Read the model definition and answer for the solid it produces. Units are mm, in the model's axes. A direction names the side the tool comes from. Give positions to 0.01 mm unless a question says otherwise; leave off trailing zeros. Loops run counter-clockwise (first coordinate to the right, second up) from the corner with the lowest first, then second, coordinate; pieces in that order, holes last. Notation, with made-up numbers: (33.25, 8.25) - (74.25, 8.25) arc R6 ccw to (74.25, 15.25) - close; hole circle Ø1 at (-20, 57.25). An arc over 180 degrees is marked (long way). Use a Markdown table: item, result. Add a question column.
Item 1: Which of the six approach directions +Z, -Z, +X, -X, +Y, -Y give full straight-line access (tool end or side, diameter ignored) to faces 1 (the face through (8, -12, -8.5)), 2 (the face through (34, -16, 0)), 3 (the face through (22, -13.75, 0)), 4 (the face through (0, 6, -10)), 5 (the face through (-32, -13.75, 0))?
Item 2: Consider probe 1 along X at (y, z) = (-16.85, 0); probe 2 along X at (y, z) = (-5.5, -2.25); probe 3 along Z at (x, y) = (6.5, 7.5). Determine where each line is inside the solid, lowest interval first. Write a range as [from, to].
Item 3: A cutting plane is placed at B-B (z = 0). Give the number of separate pieces and of enclosed holes in the cut face, plus the area to 3 significant figures.
Item 4: A cutting plane is placed at A-A (x = 6.91). Determine the outline of the cut face in (y, z) (3 decimals).
Item 5: For a pull along Z with two mould halves and no side action, classify faces 6 (the face through (0, 0, -11)), 7 (the face through (-4, -5.25, 0)), 8 (the face through (20, 2, 0)), 9 (the face through (-24.47, -16.84, -0.33)) as +Z half, -Z half, draft (parallel to the pull), parting line (faces both ways), or undercut.
Item 6: Each of these flat-tipped pins is pushed along its axis until it touches: P1, Ø10, axis at x = 5.5, y = -11, coming from the +Z side; P2, Ø1.5, axis at y = -4.5, z = -0.5, coming from the +X side; P3, Ø4.5, axis at y = -10.5, z = -0.5, coming from the -X side; P4, Ø7.5, axis at x = -29, z = 0, coming from the +Y side. Where does it stop, or does it pass through?
Item 7: A cutting plane is placed at D-D (x = -27). Determine the outline of the cut face in (y, z), plus the area to 3 significant figures.
Item 8: A cutting plane is placed at C-C (y = 14). Determine the outline of the cut face in (x, z), plus the area to 3 significant figures.
from build123d import *

# Parameters (mm, degrees)
SKETCH1_W           = 14
SKETCH1_H           = 22
SKETCH1_R           = 4.6
SKETCH1_R_2         = 2.55
SKETCH1_W_2         = 40
SKETCH1_W_3         = 12
SKETCH1_H_2         = 9.2
BOSS_EXTRUDE1_DEPTH = 17.75
CUT_EXTRUDE1_START  = -13.75
SKETCH1_5_W         = 14
SKETCH1_5_H         = 22
SKETCH1_5_R         = 4.6
SKETCH1_5_R_2       = 2.55
CUT_EXTRUDE1_DEPTH  = 31.5
CUT_EXTRUDE2_START  = -15.95
SKETCH1_6_R         = 4.6
SKETCH1_6_R_2       = 2.55
CUT_EXTRUDE2_DEPTH  = 2.2
CUT_EXTRUDE3_START  = 17.75
SKETCH1_7_W         = 12
SKETCH1_7_H         = 9.2
CUT_EXTRUDE3_DEPTH  = 23
CUT_EXTRUDE4_START  = -5.25
SKETCH1_8_W         = 12
SKETCH1_8_H         = 9.2
CUT_EXTRUDE4_DEPTH  = 9
CUT_EXTRUDE5_REACH  = 46.216
SKETCH2_R           = 2
SKETCH2_3_R         = 4.125
CUT_EXTRUDE6_DEPTH  = 2.5


with BuildPart() as part:
    # Sketch1 → Boss-Extrude1 (new, symmetric)
    # profile 1 of 7: a face of its own
    with BuildSketch(Plane(origin=(0, 0, 0), x_dir=(1, 0, 0), z_dir=(0, 1, 0))):
        with Locations((-27, 0)):
            Rectangle(SKETCH1_W, SKETCH1_H)
        with Locations((-27, 0)):
            Circle(SKETCH1_R, mode=Mode.SUBTRACT)
    # profile 2 of 7: a face of its own
    with BuildSketch(Plane(origin=(0, 0, 0), x_dir=(1, 0, 0), z_dir=(0, 1, 0))):
        with Locations((-27, 0)):
            Circle(SKETCH1_R)
        with Locations(Location((-27, 0, 0), (0, 0, 270))):
            Circle(SKETCH1_R_2, mode=Mode.SUBTRACT)
    # profile 3 of 7: a face of its own
    with BuildSketch(Plane(origin=(0, 0, 0), x_dir=(1, 0, 0), z_dir=(0, 1, 0))):
        Rectangle(SKETCH1_W_2, SKETCH1_H)
        with BuildLine():
            Line((11.854501341, -10), (-11.854501341, -10))
            ThreePointArc((-11.854501341, -10), (-18.86, 0), (-11.854501341, 10))
            Line((-11.854501341, 10), (11.854501341, 10))
            ThreePointArc((11.854501341, 10), (18.86, 0), (11.854501341, -10))
        make_face(mode=Mode.SUBTRACT)
    # profile 4 of 7: a face of its own
    with BuildSketch(Plane(origin=(0, 0, 0), x_dir=(1, 0, 0), z_dir=(0, 1, 0))):
        with BuildLine():
            ThreePointArc((11.854501341, 10), (18.86, 0), (11.854501341, -10))
            Line((11.854501341, -10), (-11.854501341, -10))
            ThreePointArc((-11.854501341, -10), (-18.86, 0), (-11.854501341, 10))
            Line((-11.854501341, 10), (11.854501341, 10))
        make_face()
        with Locations((6.92918915, 0)):
            Rectangle(SKETCH1_W_3, SKETCH1_H_2, mode=Mode.SUBTRACT)
    # profile 5 of 7: a face of its own
    with BuildSketch(Plane(origin=(0, 0, 0), x_dir=(1, 0, 0), z_dir=(0, 1, 0))):
        with Locations((6.92918915, 0)):
            Rectangle(SKETCH1_W_3, SKETCH1_H_2)
    # profile 6 of 7: a face of its own
    with BuildSketch(Plane(origin=(0, 0, 0), x_dir=(1, 0, 0), z_dir=(0, 1, 0))):
        with Locations((27, 0)):
            Rectangle(SKETCH1_W, SKETCH1_H)
        with Locations((27, 0)):
            Circle(SKETCH1_R, mode=Mode.SUBTRACT)
    # profile 7 of 7: a face of its own
    with BuildSketch(Plane(origin=(0, 0, 0), x_dir=(1, 0, 0), z_dir=(0, 1, 0))):
        with Locations((27, 0)):
            Circle(SKETCH1_R)
        with Locations(Location((27, 0, 0), (0, 0, 270))):
            Circle(SKETCH1_R_2, mode=Mode.SUBTRACT)
    extrude(amount=BOSS_EXTRUDE1_DEPTH, both=True)

    # Sketch1<5> → Cut-Extrude1 (cut)
    # profile 1 of 4: a face of its own
    with BuildSketch(Plane(origin=(0, 0, 0), x_dir=(1, 0, 0), z_dir=(0, 1, 0)).offset(CUT_EXTRUDE1_START)):
        with Locations((-27, 0)):
            Rectangle(SKETCH1_5_W, SKETCH1_5_H)
        with Locations((-27, 0)):
            Circle(SKETCH1_5_R, mode=Mode.SUBTRACT)
    # profile 2 of 4: a face of its own
    with BuildSketch(Plane(origin=(0, 0, 0), x_dir=(1, 0, 0), z_dir=(0, 1, 0)).offset(CUT_EXTRUDE1_START)):
        with Locations((27, 0)):
            Rectangle(SKETCH1_5_W, SKETCH1_5_H)
        with Locations((27, 0)):
            Circle(SKETCH1_5_R, mode=Mode.SUBTRACT)
    # profile 3 of 4: a face of its own
    with BuildSketch(Plane(origin=(0, 0, 0), x_dir=(1, 0, 0), z_dir=(0, 1, 0)).offset(CUT_EXTRUDE1_START)):
        with Locations((-27, 0)):
            Circle(SKETCH1_5_R)
        with Locations(Location((-27, 0, 0), (0, 0, 270))):
            Circle(SKETCH1_5_R_2, mode=Mode.SUBTRACT)
    # profile 4 of 4: a face of its own
    with BuildSketch(Plane(origin=(0, 0, 0), x_dir=(1, 0, 0), z_dir=(0, 1, 0)).offset(CUT_EXTRUDE1_START)):
        with Locations((27, 0)):
            Circle(SKETCH1_5_R)
        with Locations(Location((27, 0, 0), (0, 0, 270))):
            Circle(SKETCH1_5_R_2, mode=Mode.SUBTRACT)
    extrude(amount=CUT_EXTRUDE1_DEPTH, mode=Mode.SUBTRACT)

    # Sketch1<6> → Cut-Extrude2 (cut)
    # profile 1 of 2: a face of its own
    with BuildSketch(Plane(origin=(0, 0, 0), x_dir=(1, 0, 0), z_dir=(0, 1, 0)).offset(CUT_EXTRUDE2_START)):
        with Locations(Location((-27, 0, 0), (0, 0, 270))):
            Circle(SKETCH1_6_R)
        with Locations(Location((-27, 0, 0), (0, 0, 270))):
            Circle(SKETCH1_6_R_2, mode=Mode.SUBTRACT)
    # profile 2 of 2: a face of its own
    with BuildSketch(Plane(origin=(0, 0, 0), x_dir=(1, 0, 0), z_dir=(0, 1, 0)).offset(CUT_EXTRUDE2_START)):
        with Locations(Location((27, 0, 0), (0, 0, 270))):
            Circle(SKETCH1_6_R)
        with Locations(Location((27, 0, 0), (0, 0, 270))):
            Circle(SKETCH1_6_R_2, mode=Mode.SUBTRACT)
    extrude(amount=CUT_EXTRUDE2_DEPTH, mode=Mode.SUBTRACT)

    # Sketch1<7> → Cut-Extrude3 (cut)
    # profile 1 of 2: a face of its own
    with BuildSketch(Plane(origin=(0, 0, 0), x_dir=(1, 0, 0), z_dir=(0, 1, 0)).offset(CUT_EXTRUDE3_START)):
        with BuildLine():
            ThreePointArc((11.854501341, 10), (18.86, 0), (11.854501341, -10))
            Line((11.854501341, -10), (-11.854501341, -10))
            ThreePointArc((-11.854501341, -10), (-18.86, 0), (-11.854501341, 10))
            Line((-11.854501341, 10), (11.854501341, 10))
        make_face()
        with Locations((6.92918915, 0)):
            Rectangle(SKETCH1_7_W, SKETCH1_7_H, mode=Mode.SUBTRACT)
    # profile 2 of 2: a face of its own
    with BuildSketch(Plane(origin=(0, 0, 0), x_dir=(1, 0, 0), z_dir=(0, 1, 0)).offset(CUT_EXTRUDE3_START)):
        with Locations((6.92918915, 0)):
            Rectangle(SKETCH1_7_W, SKETCH1_7_H)
    extrude(amount=-CUT_EXTRUDE3_DEPTH, mode=Mode.SUBTRACT)

    # Sketch1<8> → Cut-Extrude4 (cut)
    with BuildSketch(Plane(origin=(0, 0, 0), x_dir=(1, 0, 0), z_dir=(0, 1, 0)).offset(CUT_EXTRUDE4_START)):
        with Locations((6.92918915, 0)):
            Rectangle(SKETCH1_8_W, SKETCH1_8_H)
    extrude(amount=-CUT_EXTRUDE4_DEPTH, mode=Mode.SUBTRACT)

    # Cut-Extrude5: up to this face of the body (flat: up to its plane)
    cut_extrude5_end = Plane(part.part.faces().sort_by_distance((0, -1.151436031, 11))[0])
    # Sketch2 → Cut-Extrude5 (cut, up to the picked face)
    with BuildSketch(Plane(origin=(0, 0, -11), x_dir=(-1, 0, 0), z_dir=(0, 0, -1)), mode=Mode.PRIVATE) as cut_extrude5_sk1:
        with Locations((-6.91, -9.77)):
            Circle(SKETCH2_R)
    cut_extrude5_tool1 = split(extrude(cut_extrude5_sk1.sketch, amount=-CUT_EXTRUDE5_REACH, mode=Mode.PRIVATE), bisect_by=cut_extrude5_end, keep=Keep.BOTH, mode=Mode.PRIVATE)
    add(cut_extrude5_tool1.solids().sort_by(Axis((6.91, -9.77, -11), (0, 0, 1)))[0], mode=Mode.SUBTRACT)

    # Sketch2<3> → Cut-Extrude6 (cut)
    with BuildSketch(Plane(origin=(0, 0, -11), x_dir=(-1, 0, 0), z_dir=(0, 0, -1))):
        with Locations((-6.91, -9.77)):
            Circle(SKETCH2_3_R)
    extrude(amount=-CUT_EXTRUDE6_DEPTH, mode=Mode.SUBTRACT)


solid = part.part
Geometry says:
| question | item | result |
|---|---|---|
| 1 | face 1 | -Z |
| 1 | face 2 | +Z, -Z, +X, +Y, -Y |
| 1 | face 3 | +Z, -Z, +X, +Y |
| 1 | face 4 | +Y |
| 1 | face 5 | +Z, -Z, -X, +Y |
| 2 | probe 1 | [-34, -29.55], [-24.45, 24.45], [29.55, 34] |
| 2 | probe 2 | [-20, 0.93], [12.93, 20] |
| 2 | probe 3 | [-11, -10], [10, 11] |
| 3 | separate pieces | 3 |
| 3 | enclosed holes | 0 |
| 3 | area | 498 mm² |
| 4 | outline | (-17.75, -11) - (-13.895, -11) - (-13.895, -8.5) - (-11.77, -8.5) - (-11.77, -4.6) - (-14.25, -4.6) - (-14.25, 4.6) - (-11.77, 4.6) - (-11.77, 11) - (-17.75, 11) - close; (-7.77, -8.5) - (-5.645, -8.5) - (-5.645, -11) - (17.75, -11) - (17.75, -10) - (-5.25, -10) - (-5.25, -4.6) - (-7.77, -4.6) - close; (-7.77, 4.6) - (-5.25, 4.6) - (-5.25, 10) - (17.75, 10) - (17.75, 11) - (-7.77, 11) - close |
| 5 | face 6 | -Z half |
| 5 | face 7 | undercut |
| 5 | face 8 | draft |
| 5 | face 9 | undercut |
| 6 | P1 | z = 11 |
| 6 | P2 | x = 20 |
| 6 | P3 | x = -20 |
| 6 | P4 | y = -13.75 |
| 7 | outline | (-17.75, -11) - (-13.75, -11) - (-13.75, -4.6) - (-15.95, -4.6) - (-15.95, -2.55) - (-17.75, -2.55) - close; (-17.75, 2.55) - (-15.95, 2.55) - (-15.95, 4.6) - (-13.75, 4.6) - (-13.75, 11) - (-17.75, 11) - close |
| 7 | area | 58.6 mm² |
| 8 | outline | (-20, -11) - (20, -11) - (20, 11) - (-20, 11) - close; hole (-11.85, -10) - (11.85, -10) arc R10.64 ccw to (11.85, 10) - (-11.85, 10) arc R10.64 ccw to start |
| 8 | area | 202 mm² |
